```python
from build123d import *

# Parameters (mm, degrees)
SKETCH1_R                = 0.75
BOSS_EXTRUDE1_DEPTH      = 10
BOSS_EXTRUDE2_DEPTH      = 1.5
BOSS_EXTRUDE2_DEPTH_BACK = 1.5
FILLET1_R                = 1
SKETCH3_R                = 0.6
CUT_EXTRUDE1_DEPTH       = 5


with BuildPart() as part:
    # Sketch1 → Boss-Extrude1 (new body)
    with BuildSketch(Plane(origin=(0, 0, 0), x_dir=(0, 0, -1), z_dir=(1, 0, 0))):
        Circle(SKETCH1_R)
    extrude(amount=BOSS_EXTRUDE1_DEPTH)

    # Sketch2 → Boss-Extrude2 (add, two sides: drawn at the far end of the back side and taken through both)
    with BuildSketch(Plane(origin=(0, 0, 0), x_dir=(1, 0, 0), z_dir=(0, 1, 0)).offset(-BOSS_EXTRUDE2_DEPTH_BACK)):
        Polygon((1, 1.75), (1, -1.75), (-3, -1.75), (-3, -0.75), (0, -0.75), (0, 0.75), (-3, 0.75), (-3, 1.75), align=None)
    extrude(amount=BOSS_EXTRUDE2_DEPTH + BOSS_EXTRUDE2_DEPTH_BACK)

    # Fillet1
    fillet1_edges = [part.edges().sort_by_distance(p)[0] for p in [
        (-3, 1.5, 1.25),
        (-3, 1.5, -1.25),
        (-3, -1.5, -1.25),
        (1, 0, -1.75),
        (1, 0, 1.75),
        (-3, -1.5, 1.25),
    ]]
    fillet(fillet1_edges, radius=FILLET1_R - 0.0001)  # a hair under: the kernel refuses the full size

    # Sketch3 → Cut-Extrude1 (cut)
    with BuildSketch(Plane(origin=(0, 0, -1.75), x_dir=(-1, 0, 0), z_dir=(0, 0, -1))):
        with Locations((1.7, 0)):
            Circle(SKETCH3_R)
    extrude(amount=-CUT_EXTRUDE1_DEPTH, mode=Mode.SUBTRACT)


solid = part.part
```
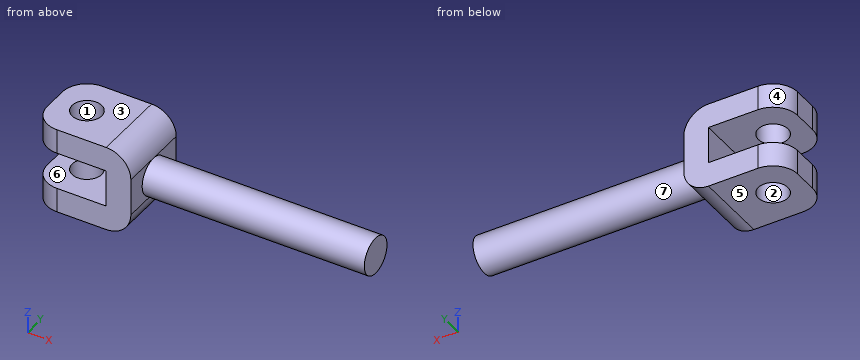
Can you work these out from the model? Positions are in its coordinate system, mm. Face numbers are marked on the shaded views. A direction names the side the tool comes from. Coordinates: 2 decimals unless noted, no trailing zeros. Loops run counter-clockwise (first coordinate to the right, second up) from the corner with the lowest first, then second, coordinate; pieces in that order, holes last.
Item 1: Suppose I cut it at C-C (z = 0). Please give me the cut outline in (x, y), then the cut area to 3 significant figures.
Answers below:
outline: (0, -1.5) - (1, -1.5) - (1, -0.75) - (10, -0.75) - (10, 0.75) - (1, 0.75) - (1, 1.5) - (0, 1.5) - close
area: 16.5 mm2
Item 2: Suppose I cut it at A-A (y = 0). State how many separate pieces and enclosed holes the cut face has, then the cut area to 3 significant figures.
Answers below:
separate pieces: 3
enclosed holes: 0
area: 20.2 mm2
Item 3: Please list where these lines run through material, in increasing order: L1, parallel to Y at x = -1.7, z = -1.25; L2, parallel to Z at x = -0.75, y = 1.15; L3, parallel to X at y = -0.45, z = 0.7.
Answers below:
L1: y = -1.5 to -0.6, 0.6 to 1.5
L2: z = -1.75 to -0.75, 0.75 to 1.75
L3: x = 0 to 1
Item 4: Which directions (+Z, -Z, +X, -X, +Y, -Y) give clear straight access to the entire face, cutting with the end or side of a thin tool? Please do the marked faces 5, 6 and 7.
Answers below:
face 5: -Z, +X, -X, +Y, -Y
face 6: -X, +Y, -Y
face 7: +X
Item 5: Suppose I cut it at D-D (z = -1.05). Please give me the cut outline in (x, y).
Answers below:
outline: (-3, -0.5) arc R1 ccw to (-2, -1.5) - (0.95, -1.5) - (0.95, 1.5) - (-2, 1.5) arc R1 ccw to (-3, 0.5) - close; hole circle Ø1.2 at (-1.7, 0)
Item 6: Suppose I cut it at B-B (x = -1.7). Please give me the cut outline in (y, z).
Answers below:
outline: (-1.5, -1.75) - (-0.6, -1.75) - (-0.6, -0.75) - (-1.5, -0.75) - close; (-1.5, 0.75) - (-0.6, 0.75) - (-0.6, 1.75) - (-1.5, 1.75) - close; (0.6, -1.75) - (1.5, -1.75) - (1.5, -0.75) - (0.6, -0.75) - close; (0.6, 0.75) - (1.5, 0.75) - (1.5, 1.75) - (0.6, 1.75) - close
Item 7: I'm going to push flat-ended pins straight in: pin 1 (1.6 mm diameter, centred on y = 0.5, z = 0, fed in from -X); pin 2 (1.5 mm diameter, centred on y = 1, z = -1.5, fed in from +X). Where does each tip first touch, or does it pass through?
Answers below:
pin 1: stops at x = -3
pin 2: stops at x = 1
Item 8: If we mould it in two halves opening along Y, with no side actions, what happens to the marked faces 1, 2, 3 and 4? For each: released by +Y, released by -Y, zero draft, split by the parting line, or undercut.
Answers below:
face 1: undercut
face 2: undercut
face 3: zero draft
face 4: released by +Y
